Autodesk Inventor part; units mm, degrees
ref_plane "YZ Plane" through (0, 0, 0) normal (1, 0, 0) x (0, 1, 0)
ref_plane "XZ Plane" through (0, 0, 0) normal (0, 1, 0) x (-1, 0, 0)
ref_plane "XY Plane" through (0, 0, 0) normal (0, 0, 1) x (1, 0, 0)
sketch "스케치1" plane through (0, 0, 0) normal (0, 1, 0) x (-1, 0, 0)
  circle A0 centre (0, 0) radius 7.5
  circle A1 centre (0, 0) radius 5.25
  dimension "d0" = 15
  dimension "d1" = 10.5
extrude "돌출1" add sketch "스케치1" against normal blind 3 contours A0 | A1
extrude "돌출2" add sketch "스케치1" along normal blind 3
sketch "스케치2" plane through (0, -3, 0) normal (0, -1, 0) x (1, 0, 0)
  circle A0 centre (0, 0) radius 5
  circle A1 centre (0, 0) radius 6
  circle A2 centre (0, 0) radius 7.5
  dimension "d6" = 10
  dimension "d7" = 12
extrude "돌출3" cut sketch "스케치2" against normal blind 0.5
properties part number "나사 회전축"
The listing builds one solid part. Answer for the finished solid, in the listing's coordinates (mm). A direction names the side the tool comes from. Coordinates: 2 decimals unless noted, no trailing zeros. Write each loop counter-clockwise with the first axis right and the second up, starting at its lowest first coordinate (ties: lowest second). Pieces come first, ordered by that corner, then holes. Notation, with made-up numbers: (-39.75, -34.5) - (6.25, -34.5) arc R29 cw to (6.25, -12.5) - close; hole circle Ø5 at (20.25, -8.75). An arc over 180 degrees is marked (long way). Return JSON: item names as keys, results as strings. Group by question number.
1. A cutting plane is placed at C-C, the plane y = 1.8. Determine the outline of the cut face in (x, z), plus the area to 3 significant figures.
2. A cutting plane is placed at D-D, the plane y = -0.35. Determine the outline of the cut face in (x, z), plus the area to 3 significant figures.
3. A cutting plane is placed at B-B, the plane z = 0. Determine the outline of the cut face in (x, y).
4. Given pin 1 (9 mm diameter, centred on x = 0, z = 0, fed in from +Y); pin 2 (3 mm diameter, centred on x = 1.5, z = -1.5, fed in from -Y); pin 3 (1.5 mm diameter, centred on y = -2.5, z = -1, fed in from -X), each flat-ended and moving along its own axis, determine where each tip first touches the part or whether it passes through.
5. Determine the mould class of faces 1 (the cylindrical face through (-5.994, -2.754, 0.264)), 2 (the flat face through (4, -3, 4)), 3 (the cylindrical face through (-5, 1.5, -1.6)) for opening direction Z: released by +Z, released by -Z, zero draft, split by the parting line, or undercut.
6. Straight lines are drawn through the part: L1, parallel to Z at x = 0, y = 2; L2, parallel to Z at x = 0, y = -2.6; L3, parallel to Y at x = -4.25, z = -2. For each, find the intervals that lie inside material, in ascending order.
7. Which of the six approach directions +Z, -Z, +X, -X, +Y, -Y give full straight-line access (tool end or side, diameter ignored) to faces 4 (the flat face through (0, 0, 0)), 5 (the flat face through (0, -2.5, 0)), 6 (the flat face through (1.8, 3, 5.1))?
8. A cutting plane is placed at A-A, the plane x = 0. Determine the outline of the cut face in (y, z), plus the area to 3 significant figures.
Ans:
{
 "1": {"outline": "circle Ø15 at (0, 0); hole circle Ø10.5 at (0, 0)", "area": "90.1 mm²"},
 "2": {"outline": "circle Ø15 at (0, 0)", "area": "177 mm²"},
 "3": {"outline": "(-7.5, -2.5) - (-6, -2.5) - (-6, -3) - (-5, -3) - (-5, -2.5) - (5, -2.5) - (5, -3) - (6, -3) - (6, -2.5) - (7.5, -2.5) - (7.5, 3) - (5.25, 3) - (5.25, 0) - (-5.25, 0) - (-5.25, 3) - (-7.5, 3) - close"},
 "4": {"pin 1": "y = 0", "pin 2": "y = -2.5", "pin 3": "x = -7.5"},
 "5": {"face 1": "split by the parting line", "face 2": "zero draft", "face 3": "undercut"},
 "6": {"L1": "-7.5 to -5.25, 5.25 to 7.5", "L2": "-6 to -5, 5 to 6", "L3": "-2.5 to 0"},
 "7": {"face 4": "+Y", "face 5": "-Y", "face 6": "+Z, -Z, +X, -X, +Y"},
 "8": {"outline": "(-3, -6) - (-2.5, -6) - (-2.5, -7.5) - (3, -7.5) - (3, -5.25) - (0, -5.25) - (0, 5.25) - (3, 5.25) - (3, 7.5) - (-2.5, 7.5) - (-2.5, 6) - (-3, 6) - (-3, 5) - (-2.5, 5) - (-2.5, -5) - (-3, -5) - close", "area": "52.0 mm²"}
}
